For this review, take the finished solid that the model builds, in its own axes (mm). Face numbers are marked on the shaded views. A direction names the side the tool comes from. Round coordinates to 2 decimals unless told otherwise and drop trailing zeros. Loops run counter-clockwise (first coordinate to the right, second up) from the corner with the lowest first, then second, coordinate; pieces in that order, holes last.
1. Consider section C-C on y = 62.5. State the section outline as (x, z) points.
2. Clearance check with flat-ended pins moving along their axes: pin 1 Ø4 at (y, z) = (74, -64.5) entering from -X; pin 2 Ø5 at (x, z) = (120, -37) entering from +Y; pin 3 Ø3 at (y, z) = (95, 83) entering from -X. State where each tip first meets the part, or that it passes through.
3. Consider section B-B on x = -341.5. State the section outline as (y, z) points.
4. Draft analysis for pull direction Z (two halves, no side actions). For the marked faces 4, 5 and 6, state which applies: released by +Z, released by -Z, zero draft, split by the parting line, or undercut.
5. Tool access review of the marked faces 1, 2 and 3: name each direction out of +Z, -Z, +X, -X, +Y, -Y from which nothing blocks a thin tool from reaching the whole face with its end or side.
6. Consider section A-A on z = 249. State the section outline as (x, y) points.
7. To check wall thickness, follow line 1 along Z through (x, y) = (-226, 96); line 2 along Y through (x, z) = (-226.5, 234); line 3 along Z through (x, y) = (209, 68). State the ranges of each line that lie inside material, in increasing order.
8. Consider section D-D on y = -87.5. State how many separate pieces and enclosed holes the cut face has, then the cut area to 3 significant figures.
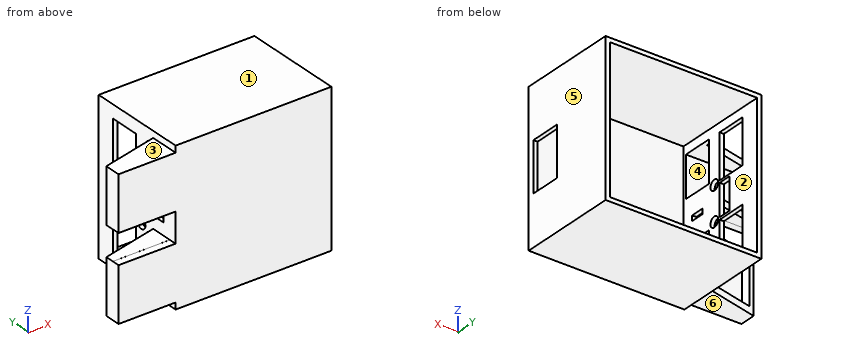
from build123d import *

# Parameters (mm, degrees)
F0_W      = 475
F0_H      = 310
F1_DEPTH  = 115
F2_T      = -12.7
F3_W      = 93
F3_H      = 125
F3_H_2    = 135
F4_DEPTH  = 25
F5_DEPTH  = 25
F7_DEPTH  = 174
F8_W      = 15
F8_H      = 125
F10_DEPTH = 35
F11_DEPTH = 363
F13_W     = 42.5
F13_H     = 7.8922572035
F13_W_2   = 40
F13_H_2   = 48.3056434989
F13_H_3   = 48.6943565011
F13_H_4   = 8.1077427965
F14_DEPTH = 25
F15_W     = 95
F15_H     = 150
F16_DEPTH = 25
F13_R     = 15.5
F17_DEPTH = 25


# Not quite as in the source:
# - a feature names something its author has since deleted; it is built from what else it names


with BuildPart() as f1:
    # F0 (on Top) → F1 (new body, symmetric)
    with BuildSketch(Plane.XY):
        Rectangle(F0_W, F0_H)
    extrude(amount=F1_DEPTH, both=True)

    # F2
    f2_openings = [f1.faces().sort_by_distance(p)[0] for p in [
        (0, 0, 115),
    ]]
    offset(amount=F2_T, openings=f2_openings)

    # F3 (on face) → F4 (cut)
    with BuildSketch(Plane(origin=(-237.5, 0, 0), x_dir=(0, -1, 0), z_dir=(-1, 0, 0))):
        with Locations((85.4776808544, -12.5305280089)):
            Rectangle(F3_W, F3_H)
        with Locations((-50.0830374043, -7.5305280089)):
            Rectangle(F3_W, F3_H_2)
    extrude(amount=-F4_DEPTH, mode=Mode.SUBTRACT)

    # F5 (cut): a face of the model
    f5_faces = [f1.faces().sort_by_distance(p)[0] for p in [
        (0, 142.3, 6.35),
    ]]
    extrude(f5_faces, amount=-F5_DEPTH, mode=Mode.SUBTRACT)

    # F6 (on face) → F7 (join)
    with BuildSketch(Plane(origin=(-237.5, 0, 0), x_dir=(0, -1, 0), z_dir=(-1, 0, 0))):
        Polygon((131.9776808544, -75.0305280089), (38.9776808544, -75.0305280089), (38.9776808544, -95.0305280089), (131.9776808544, -95.0305280089), (155, -95.0305280089), (155, 69.9025020003), (131.9776808544, 69.9025020003), (131.9776808544, 69.9694719911), (38.9776808544, 69.9694719911), (38.9776808544, 49.9694719911), (131.9776808544, 49.9694719911), align=None)
    extrude(amount=F7_DEPTH)

    # F8 (on face) → F10 (join)
    with BuildSketch(Plane(origin=(0, -131.9776808544, 0), x_dir=(-1, 0, 0), z_dir=(0, 1, 0))):
        with Locations((404, -12.5305280089)):
            Rectangle(F8_W, F8_H)
    extrude(amount=F10_DEPTH)

    # F9 (on face) → F11 (cut)
    with BuildSketch(Plane(origin=(0, 0, -95.0305280089), x_dir=(1, 0, 0), z_dir=(0, 0, -1))):
        Polygon((-411.5, 38.9776808544), (-237.5, 38.9776808544), (-237.5, 64.5424127579), (-411.5, 105.7684645057), align=None)
    extrude(amount=-F11_DEPTH, mode=Mode.SUBTRACT)

    # F12: F1 across face


with BuildPart() as f1_1:
    add(f1.part)
    add(f1.part.mirror(Plane(origin=(0, -62.4841436051, 115), x_dir=(1, 0, 0), z_dir=(0, 0, 1))))

    # F13 (on face) → F14 (cut)
    with BuildSketch(Plane(origin=(-237.5, 0, 0), x_dir=(0, -1, 0), z_dir=(-1, 0, 0))):
        with Locations((85.7924127579, 118.9461286017)):
            Rectangle(F13_W, F13_H)
        with Locations((-23.5830374043, 90.8471782506)):
            Rectangle(F13_W_2, F13_H_2)
        with Locations((-23.5830374043, 139.3471782506)):
            Rectangle(F13_W_2, F13_H_3)
        with Locations((85.7924127579, 110.9461286017)):
            Rectangle(F13_W, F13_H_4)
    extrude(amount=-F14_DEPTH, mode=Mode.SUBTRACT)

    # F15 (on face) → F16 (cut)
    with BuildSketch(Plane.YZ.offset(237.5)):
        with Locations((-88.2316343486, 111.4078534107)):
            Rectangle(F15_W, F15_H)
    extrude(amount=-F16_DEPTH, mode=Mode.SUBTRACT)

    # F13 (on face) → F17 (cut)
    with BuildSketch(Plane(origin=(-237.5, 0, 0), x_dir=(0, -1, 0), z_dir=(-1, 0, 0))):
        with Locations((17.697321725, 166.6680857539)):
            Circle(F13_R)
        with BuildLine():
            ThreePointArc((33.197321725, 63.3319142461), (17.697321725, 78.8319142461), (2.197321725, 63.3319142461))
            Line((2.197321725, 63.3319142461), (17.697321725, 63.3319142461))
            Line((17.697321725, 63.3319142461), (33.197321725, 63.3319142461))
        make_face()
        with BuildLine():
            Line((17.697321725, 63.3319142461), (2.197321725, 63.3319142461))
            ThreePointArc((2.197321725, 63.3319142461), (17.697321725, 47.8319142461), (33.197321725, 63.3319142461))
            Line((33.197321725, 63.3319142461), (17.697321725, 63.3319142461))
        make_face()
    extrude(amount=-F17_DEPTH, mode=Mode.SUBTRACT)


solid = f1_1.part
Resolved:
1. outline: (-237.5, -115) - (237.5, -115) - (237.5, 345) - (-237.5, 345) - (-237.5, 305.03) - (-224.8, 305.03) - (-224.8, 332.3) - (224.8, 332.3) - (224.8, -102.3) - (-224.8, -102.3) - (-224.8, -75.03) - (-237.5, -75.03) - close; (-237.5, 59.97) - (-224.8, 59.97) - (-224.8, 170.03) - (-237.5, 170.03) - close
2. pin 1: stops at x = 224.8
2. pin 2: stops at y = -142.3
2. pin 3: stops at x = -237.5
3. outline: (-155, -95.03) - (-89.18, -95.03) - (-89.18, -75.03) - (-131.98, -75.03) - (-131.98, 49.97) - (-89.18, 49.97) - (-89.18, 69.97) - (-131.98, 69.97) - (-131.98, 69.9) - (-155, 69.9) - close; (-155, 160.1) - (-131.98, 160.1) - (-131.98, 160.03) - (-89.18, 160.03) - (-89.18, 180.03) - (-131.98, 180.03) - (-131.98, 305.03) - (-89.18, 305.03) - (-89.18, 325.03) - (-155, 325.03) - close
4. face 4: undercut
4. face 5: zero draft
4. face 6: released by -Z
5. face 1: +Z, +X, -X, +Y, -Y
5. face 2: +Y
5. face 3: +Z, -X, +Y, -Y
6. outline: (-411.5, -155) - (237.5, -155) - (237.5, 155) - (224.8, 155) - (224.8, -142.3) - (-224.8, -142.3) - (-224.8, -131.98) - (-396.5, -131.98) - (-396.5, -102.21) - (-411.5, -105.77) - close; (-237.5, -38.98) - (-224.8, -38.98) - (-224.8, 3.58) - (-237.5, 3.58) - close; (-237.5, 96.58) - (-224.8, 96.58) - (-224.8, 155) - (-237.5, 155) - close
7. line 1: z = -115 to -75.03, 59.97 to 170.03, 305.03 to 345
7. line 2: y = -155 to -131.98, -38.98 to 3.58, 96.58 to 155
7. line 3: z = -115 to -102.3, 332.3 to 345
8. separate pieces: 4
8. enclosed holes: 0
8. area: 25,600 mm2
